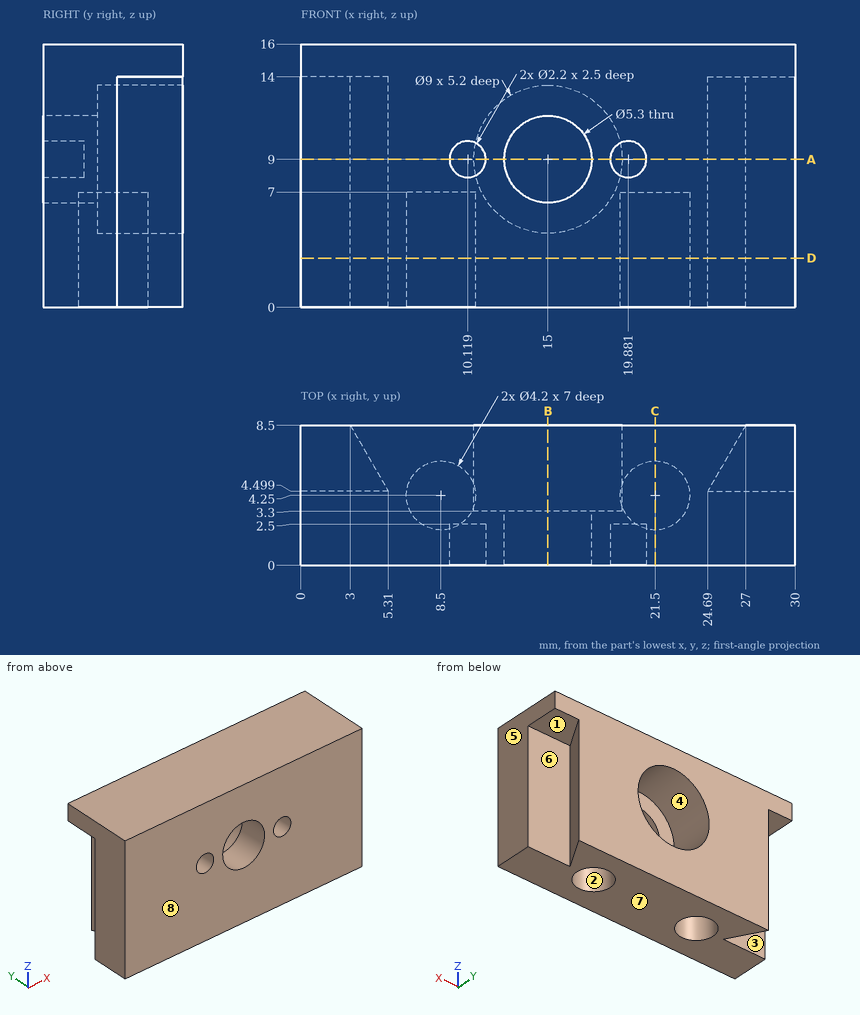
Check sheet for the drawn part. Datum: minimum x, y, z corner. Units: mm. A direction names the side the tool comes from. Round coordinates to 2 decimals unless told otherwise and drop trailing zeros. Order: outer loops, then holes, each group sorted by start corner. A loop starts at its lowest first (then second) coordinate and runs counter-clockwise, first axis right, second up. Notation, with made-up numbers: (54.5, 82) - (111.5, 82) arc R9 cw to (111.5, 86) - close; hole circle Ø3 at (74, -36.75). An arc over 180 degrees is marked (long way). Use a Markdown table: item, result. Add a question column.
(1) Sectioned sample at C-C, the plane x = 21.5. Enter the section's corners in (y, z).
(2) Depth check by flat-ended pin: pin 1 (2 mm diameter, centred on x = 27.5, y = 6, fed in from -Z); pin 2 (5 mm diameter, centred on x = 15, z = 9, fed in from -Y); pin 3 (1.6 mm diameter, centred on x = 1.5, z = 10, fed in from +Y); pin 4 (1.1 mm diameter, centred on x = 20, z = 9, fed in from -Y). Enter the tip coordinate at first touch or a pass-through.
(3) Sectioned sample at B-B, the plane x = 15. Enter the section's corners in (y, z).
(4) Tool access check on the marked faces 1, 2, 3, 4 and 5. Record the directions out of +Z, -Z, +X, -X, +Y, -Y that give a thin tool (end or side, any length) a straight path to the whole face; none if there is none.
(5) Material ranges on line 1 along X through (y, z) = (1.65, 9); line 2 along Z through (x, y) = (10, 2.25); line 3 along Y through (x, z) = (21.5, 5.75), recorded low to high. Write a range as [from, to].
(6) Sectioned sample at A-A, the plane z = 9. Enter the section's corners in (x, y).
(7) Sectioned sample at D-D, the plane z = 3. Enter the section's corners in (x, y), and give its area (3 significant figures).
(8) Release check for a two-part mould opening along Y. For the marked faces 6, 7 and 8 record: pulls with the +Y half, pulls with the -Y half, needs draft (parallel to the pull), parting line crosses it, or undercut.
Answers below:
| question | item | result |
|---|---|---|
| 1 | outline | (0, 0) - (2.15, 0) - (2.15, 7) - (6.35, 7) - (6.35, 0) - (8.5, 0) - (8.5, 16) - (0, 16) - close |
| 2 | pin 1 | z = 14 |
| 2 | pin 2 | through |
| 2 | pin 3 | y = 4.5 |
| 2 | pin 4 | y = 2.5 |
| 3 | outline | (0, 0) - (8.5, 0) - (8.5, 4.5) - (3.3, 4.5) - (3.3, 6.35) - (0, 6.35) - close; (0, 11.65) - (3.3, 11.65) - (3.3, 13.5) - (8.5, 13.5) - (8.5, 16) - (0, 16) - close |
| 4 | face 1 | -Z, +X |
| 4 | face 2 | -Z |
| 4 | face 3 | -Z, -X |
| 4 | face 4 | +Y |
| 4 | face 5 | +Z, -Z, +X, +Y, -Y |
| 5 | line 1 | [0, 9.02], [11.22, 12.35], [17.65, 18.78], [20.98, 30] |
| 5 | line 2 | [0, 7.91], [10.09, 16] |
| 5 | line 3 | [0, 2.15], [6.35, 8.5] |
| 6 | outline | (0, 0) - (9.02, 0) - (9.02, 2.5) - (11.22, 2.5) - (11.22, 0) - (12.35, 0) - (12.35, 3.3) - (10.5, 3.3) - (10.5, 8.5) - (3, 8.5) - (5.31, 4.5) - (0, 4.5) - close; (17.65, 0) - (18.78, 0) - (18.78, 2.5) - (20.98, 2.5) - (20.98, 0) - (30, 0) - (30, 4.5) - (24.69, 4.5) - (27, 8.5) - (19.5, 8.5) - (19.5, 3.3) - (17.65, 3.3) - close |
| 7 | outline | (0, 0) - (30, 0) - (30, 4.5) - (24.69, 4.5) - (27, 8.5) - (3, 8.5) - (5.31, 4.5) - (0, 4.5) - close; hole circle Ø4.2 at (8.5, 4.25); hole circle Ø4.2 at (21.5, 4.25) |
| 7 | area | 194 mm² |
| 8 | face 6 | undercut |
| 8 | face 7 | needs draft |
| 8 | face 8 | pulls with the -Y half |
